Read the model definition and answer for the solid it produces. Units are mm, in the model's axes. Face numbers are marked on the shaded views. Give positions to 0.01 mm unless a question says otherwise; leave off trailing zeros. Order: outer loops, then holes, each group sorted by start corner. A loop starts at its lowest first (then second) coordinate and runs counter-clockwise, first axis right, second up. Notation, with made-up numbers: (3, -26.75) - (27, -26.75) arc R19 cw to (27, -21.75) - close; hole circle Ø10 at (42.5, 30.5). An arc over 180 degrees is marked (long way). Write each question's results on one line, items separated by ' | '.
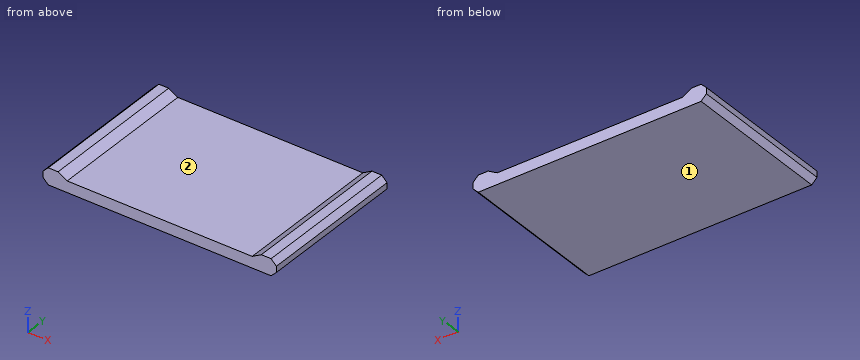
from build123d import *

# Parameters (mm, degrees)
PAD006_DEPTH = 10


with BuildPart() as part:
    # Sketch019 → Pad006 (new body, symmetric)
    with BuildSketch(Plane.XZ):
        Polygon((-39.762436, 0), (-38.55, 0.7), (-37.25, 0.7), (-36.55, 0), (-36.55, -0.8), (-37.25, -1.5), (-66.85, -1.5), (-67.55, -0.8), (-67.55, 0), (-66.85, 0.7), (-65.55, 0.7), (-64.337564, 0), align=None)
    extrude(amount=PAD006_DEPTH, both=True)


solid = part.part
(1) This flat-tipped pin is pushed along its axis until it touches: pin 1 (6 mm diameter, centred on x = -48, y = -1, fed in from +Z). Where does it stop, or does it pass through?
Conclusion:
pin 1: z = 0
(2) The mould has two halves that part along X. Classify the marked faces 1 and 2: pulls with the +X half, pulls with the -X half, needs draft (parallel to the pull), parting line crosses it, or undercut.
Conclusion:
face 1: needs draft | face 2: undercut
(3) Section C-C (z = -1.15) is taken. Give the vertices of the cut face in (x, y), plus the area to 3 significant figures.
Conclusion:
outline: (-67.2, -10) - (-36.9, -10) - (-36.9, 10) - (-67.2, 10) - close | area: 606 mm^2
(4) Consider probe 1 along Z at (x, y) = (-61, -1.75); probe 2 along X at (y, z) = (8, 0.05); probe 3 along X at (y, z) = (-7, 0.6). Determine where each line is inside the solid, lowest interval first. Write a range as [from, to].
Conclusion:
probe 1: [-1.5, 0] | probe 2: [-67.5, -64.42], [-39.68, -36.6] | probe 3: [-66.95, -65.38], [-38.72, -37.15]
(5) Section A-A (y = 8.5) is taken. Give the vertices of the cut face in (x, z), plus the area to 3 significant figures.
Conclusion:
outline: (-67.55, -0.8) - (-66.85, -1.5) - (-37.25, -1.5) - (-36.55, -0.8) - (-36.55, 0) - (-37.25, 0.7) - (-38.55, 0.7) - (-39.76, 0) - (-64.34, 0) - (-65.55, 0.7) - (-66.85, 0.7) - (-67.55, 0) - close | area: 49.2 mm^2
(6) Section B-B (x = -54.5) is taken. Give the vertices of the cut face in (y, z), plus the area to 3 significant figures.
Conclusion:
outline: (-10, -1.5) - (10, -1.5) - (10, 0) - (-10, 0) - close | area: 30.0 mm^2
